Source: CAD feature listing. Evaluate the final solid. Frame: model axes, mm. A direction names the side the tool comes from. Round coordinates to 2 decimals unless told otherwise and drop trailing zeros. Write each loop counter-clockwise with the first axis right and the second up, starting at its lowest first coordinate (ties: lowest second). Pieces come first, ordered by that corner, then holes. Notation, with made-up numbers: M 48,88.5 L 106,88.5 A27 cw 106,105.5 Z; hole C 82,39 d2. An arc over 180 degrees is marked long. Answer in a Markdown table with one row per item.
from build123d import *

# Parameters (mm, degrees)
SKETCH1_R             = 4.15
BOSS_EXTRUDE1_DEPTH   = 5
SKETCH2_R             = 2.425
BOSS_EXTRUDE2_DEPTH   = 40
CUT_EXTRUDE1_DEPTH    = 3
CHAMFER1_SIZE         = 0.5
CHAMFER1_SIZE2        = 0.419549816
CHAMFER1_PART_2_SIZE  = 0.5
CHAMFER1_PART_2_SIZE2 = 0.419549816


with BuildPart() as part:
    # Sketch1 → Boss-Extrude1 (new body)
    with BuildSketch(Plane(origin=(0, 0, 0), x_dir=(1, 0, 0), z_dir=(0, 1, 0))):
        Circle(SKETCH1_R)
    extrude(amount=BOSS_EXTRUDE1_DEPTH)

    # Sketch2 → Boss-Extrude2 (add)
    with BuildSketch(Plane(origin=(0, 5, 0), x_dir=(1, 0, 0), z_dir=(0, 1, 0))):
        Circle(SKETCH2_R)
    extrude(amount=BOSS_EXTRUDE2_DEPTH)

    # Sketch3 → Cut-Extrude1 (cut)
    with BuildSketch(Plane.XZ):
        Polygon((0, 2.786041865), (-2.412783031, 1.393020932), (-2.412783031, -1.393020932), (0, -2.786041865), (2.412783031, -1.393020932), (2.412783031, 1.393020932), align=None)
    extrude(amount=-CUT_EXTRUDE1_DEPTH, mode=Mode.SUBTRACT)

    # Chamfer1
    chamfer1_edges = [part.edges().sort_by_distance(p)[0] for p in [
        (-4.15, 0, 0),
    ]]
    chamfer1_side = [part.faces().sort_by_distance(p)[0] for p in [
        (-4.032620274, 0, 0),
    ]]
    chamfer(chamfer1_edges, length=CHAMFER1_SIZE, length2=CHAMFER1_SIZE2, reference=chamfer1_side[0])

    # Chamfer1 part 2
    chamfer1_part_2_edges = [part.edges().sort_by_distance(p)[0] for p in [
        (-4.15, 5, 0),
    ]]
    chamfer1_part_2_side = [part.faces().sort_by_distance(p)[0] for p in [
        (-4.15, 2.5, 0),
    ]]
    chamfer(chamfer1_part_2_edges, length=CHAMFER1_PART_2_SIZE, length2=CHAMFER1_PART_2_SIZE2, reference=chamfer1_part_2_side[0])


solid = part.part
Q1. Contact query for flat-ended pins moving along their axis: pin 1 Ø0.8 at (y, z) = (1.5, 0.5) entering from -X; pin 2 Ø1.4 at (x, z) = (1, -0.5) entering from -Y; pin 3 Ø1 at (y, z) = (30, -1) entering from +X. Output: stop coordinate, or through.
Solutions:
| item | result |
|---|---|
| pin 1 | stops at x = -4.15 |
| pin 2 | stops at y = 3 |
| pin 3 | stops at x = 2.37 |
Q2. Access query for faces 1 (the flat face through (-0.9, 0, -2.5)), 2 (the flat face through (-0.88, 5, 2.43)), 3 (the flat face through (-1.19, 1.48, 2.1)). Directions: +Z, -Z, +X, -X, +Y, -Y. A direction counts if a zero-diameter tool reaches every point of the face in a straight line with its end or side. Return the directions, or none.
Solutions:
| item | result |
|---|---|
| face 1 | +Z, -Z, +X, -X, -Y |
| face 2 | +Y |
| face 3 | -Y |
Q3. Section A-A (z = 0). Return loops of the section in (x, y) (3 decimals).
Solutions:
| item | result |
|---|---|
| outline | M -4.15,0.42 L -3.65,0 L -2.413,0 L -2.413,3 L 2.413,3 L 2.413,0 L 3.65,0 L 4.15,0.42 L 4.15,4.5 L 3.73,5 L 2.425,5 L 2.425,45 L -2.425,45 L -2.425,5 L -3.73,5 L -4.15,4.5 Z |
Q4. Material intervals for probe 1 along Y at (x, z) = (-2.75, 2); probe 2 along Z at (x, y) = (0, 37.5) (3 decimals); probe 3 along X at (y, z) = (25.5, -0.25), sorted ascending.
Solutions:
| item | result |
|---|---|
| probe 1 | y = 0 to 5 |
| probe 2 | z = -2.425 to 2.425 |
| probe 3 | x = -2.41 to 2.41 |
Q5. Pull-direction query (Z, two-part tool) for faces 4 (the flat face through (0, 3, 0)), 5 (the cylindrical face through (-0.9, 2.43, 4.05)), 6 (the flat face through (-2.413, 1, 0)), 7 (the flat face through (0, 45, 0)); classes: pulls with the +Z half, pulls with the -Z half, needs draft (parallel to the pull), parting line crosses it, or undercut.
Solutions:
| item | result |
|---|---|
| face 4 | undercut |
| face 5 | parting line crosses it |
| face 6 | undercut |
| face 7 | needs draft |
Q6. Section B-B (y = 39.5). Return loops of the section in (x, z) (3 decimals).
Solutions:
| item | result |
|---|---|
| outline | C 0,0 d4.85 |
